```python
from build123d import *

# Parameters (mm, degrees)
F0_R     = 10
F1_DEPTH = 10


with BuildPart() as f1:
    # F0 (on Right) → F1 (new body)
    with BuildSketch(Plane.YZ):
        with BuildLine():
            ThreePointArc((38.113879, 44.964413), (21.513052, 30.293265), (0, 25))
            ThreePointArc((0, 25), (-20.58691, 14.183763), (-23.359988, -8.905671))
            ThreePointArc((-23.359988, -8.905671), (-23.349868, -8.932169), (-23.339719, -8.958656))
            ThreePointArc((-23.339719, -8.958656), (-8.349163, -32.524314), (14.636825, -48.389412))
            ThreePointArc((14.636825, -48.389412), (38.522419, -41.970049), (37.904534, -17.244596))
            ThreePointArc((37.904534, -17.244596), (36.990811, -9.071889), (44.120823, -4.974213))
            ThreePointArc((44.120823, -4.974213), (51.812387, -3.363809), (57.634222, 1.91443))
            ThreePointArc((57.634222, 1.91443), (64.999302, 16.147055), (69.64331, 31.48476))
            ThreePointArc((69.64331, 31.48476), (59.379374, 51.091122), (38.113879, 44.964413))
        make_face()
        Circle(F0_R, mode=Mode.SUBTRACT)
        with Locations((22.5, -30)):
            Circle(F0_R, mode=Mode.SUBTRACT)
        with Locations((52.5, 35)):
            Circle(F0_R, mode=Mode.SUBTRACT)
    extrude(amount=F1_DEPTH)


solid = f1.part
```
Input: part model. Units: mm. Frame: model coordinates. Coordinates: 2 decimals unless noted, no trailing zeros. Loops run counter-clockwise (first coordinate to the right, second up) from the corner with the lowest first, then second, coordinate; pieces in that order, holes last. Notation, with made-up numbers: M -32.75,80.5 L 23.25,80.5 A22 ccw 23.25,89.5 Z; hole C 12,21 d6. An arc over 180 degrees is marked long. Use a Markdown table: item, result. Add a question column.
1) Section A-A, the plane y = 26. Return the cut outline in (x, z).
2) Draft query along Z for faces 1 (the cylindrical face through (4.93, -2.17, -9.76)), 2 (the cylindrical face through (4.93, -8.62, -32.24)), 3 (the cylindrical face through (4.93, 21.79, 30.44)). Return one class per face: +Z half, -Z half, draft (parallel to the pull), parting line (faces both ways), or undercut.
3) Section B-B, the plane z = -30. Return the cut outline in (x, y).
4) Section C-C, the plane x = 2.5. Return the cut outline in (y, z).
5) Pin query (flat end, axial travel): P1, Ø4, axis at x = 8, y = 59, coming from the -Z side; P2, Ø1, axis at x = 9, y = 15, coming from the +Z side; P3, Ø12, axis at y = 52.5, z = 35, coming from the +X side; P4, Ø5, axis at x = 4.5, y = 31, coming from the +Z side. Return the tip coordinate at first contact, or that it passes through.
6) Line query: L1, parallel to Z at x = 4.5, y = 22.5; L2, parallel to Y at x = 8, z = -37.5; L3, parallel to Y at x = 8.75, z = -8. Output: solid intervals per line, ascending. Write a range as from..to.
Answer below:
| question | item | result |
|---|---|---|
| 1 | outline | M 0,-49.69 L 10,-49.69 L 10,-39.37 L 0,-39.37 Z; M 0,-20.63 L 10,-20.63 L 10,32.98 L 0,32.98 Z |
| 2 | face 1 | undercut |
| 2 | face 2 | -Z half |
| 2 | face 3 | +Z half |
| 3 | outline | M 0,-10.66 L 10,-10.66 L 10,12.5 L 0,12.5 Z; M 0,32.5 L 10,32.5 L 10,42.5 L 0,42.5 Z |
| 4 | outline | M -23.36,-8.91 A25.94 ccw -23.34,-8.96 A70.27 ccw 14.64,-48.39 A20 ccw 37.9,-17.24 A7.5 cw 44.12,-4.97 A15 ccw 57.63,1.91 A87.44 ccw 69.64,31.48 A17.5 ccw 38.11,44.96 A46.36 cw 0,25 A25 ccw Z; hole C 0,0 d20; hole C 22.5,-30 d20; hole C 52.5,35 d20 |
| 5 | P1 | z = 1 |
| 5 | P2 | z = 27.67 |
| 5 | P3 | through |
| 5 | P4 | z = 39.31 |
| 6 | L1 | -50..-40, -20..30.83 |
| 6 | L2 | -3.03..15.89, 29.11..41.04 |
| 6 | L3 | -23.69..-6, 6..37.65 |
